Could you check a few things on this model? Use its own coordinates, in mm. Face numbers are marked on the shaded views. A direction names the side the tool comes from. Give positions to 0.01 mm unless a question says otherwise; leave off trailing zeros. Order: outer loops, then holes, each group sorted by start corner. A loop starts at its lowest first (then second) coordinate and runs counter-clockwise, first axis right, second up. Notation, with made-up numbers: M 88,24.5 L 134,24.5 A32 ccw 134,50.5 Z; hole C 73,52.5 d11. An arc over 180 degrees is marked long. Return JSON: item names as keys, results as strings. Group by question number.
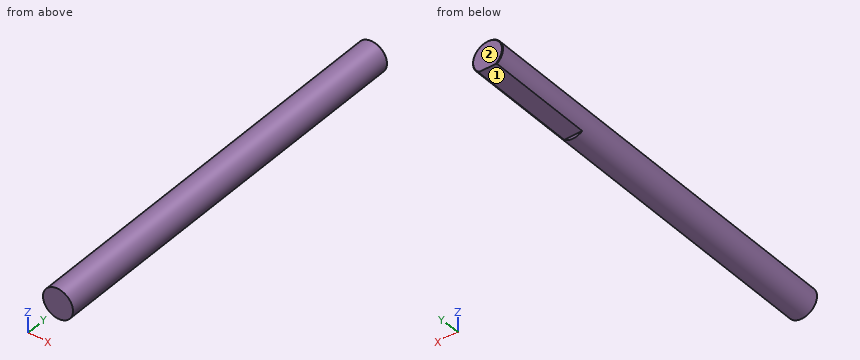
```python
from build123d import *

# Parameters (mm, degrees)
SKETCH_1_R          = 2.5
EXTRUDE_1_DEPTH     = 66
CHAMFER_1_SIZE      = 0.1
CUT_EXTRUDE_START   = -18
CUT_EXTRUDE_2_DEPTH = 18


with BuildPart() as part:
    # 草图1 → 凸台-拉伸1 (new body)
    with BuildSketch(Plane(origin=(0, 0, 0), x_dir=(1, 0, 0), z_dir=(0, 1, 0))):
        with Locations(Location((0, 0, 0), (0, 0, 270))):
            Circle(SKETCH_1_R)
    extrude(amount=EXTRUDE_1_DEPTH)

    # 倒角1
    chamfer_1_edges = [part.edges().sort_by_distance(p)[0] for p in [
        (0, 66, -2.5),
    ]]
    chamfer(chamfer_1_edges, length=CHAMFER_1_SIZE)

    # 草图2 → 切除-拉伸2 (cut)
    with BuildSketch(Plane(origin=(0, 66, 0), x_dir=(1, 0, 0), z_dir=(0, 1, 0)).offset(CUT_EXTRUDE_START)):
        with BuildLine():
            Line((-1.5, 2), (1.5, 2))
            ThreePointArc((1.5, 2), (0, 2.5), (-1.5, 2))
        make_face()
    extrude(amount=CUT_EXTRUDE_2_DEPTH, mode=Mode.SUBTRACT)


solid = part.part
```
1. Imagine slicing it at C-C, the plane y = 53.5. Please give me the cut outline in (x, z), plus the area to 3 significant figures.
2. I need wall thicknesses on L1, parallel to X at y = 53, z = -0.7; L2, parallel to X at y = 17.5, z = -0.2. Which ranges of each line are inside material? Lowest first, please. Write a range as from..to.
3. Imagine slicing it at B-B, the plane y = 36.5. Please give me the cut outline in (x, z).
4. For pin 1 (3 mm diameter, centred on y = 30, z = 1.5, fed in from -X); pin 2 (2 mm diameter, centred on y = 14, z = -1.5, fed in from +X); pin 3 (0.5 mm diameter, centred on x = -0.5, z = -2.5, fed in from +Y); pin 4 (1.5 mm diameter, centred on x = 0, y = 59, fed in from -Z), each with a flat end and sliding along its axis, tell me the tip position at first contact or that it passes through.
5. Which directions (+Z, -Z, +X, -X, +Y, -Y) give clear straight access to the entire face, cutting with the end or side of a thin tool? Please do the marked faces 1 and 2.
6. Imagine slicing it at A-A, the plane x = 0. Please give me the cut outline in (y, z).
Values:
{
 "1": {"outline": "M -1.5,-2 L 1.5,-2 A2.5 ccw long Z", "area": "18.6 mm²"},
 "2": {"L1": "x = -2.4..2.4", "L2": "x = -2.49..2.49"},
 "3": {"outline": "C 0,0 d5"},
 "4": {"pin 1": "stops at x = -2.5", "pin 2": "stops at x = 2.45", "pin 3": "stops at y = 48", "pin 4": "stops at z = -2"},
 "5": {"face 1": "-Z, +X, -X, +Y", "face 2": "+Z, -Z, +X, -X, +Y"},
 "6": {"outline": "M 0,-2.5 L 48,-2.5 L 48,-2 L 66,-2 L 66,2.4 L 65.9,2.5 L 0,2.5 Z"}
}
